Work out the finished part from the listing and answer in its coordinate system (mm). Face numbers are marked on the shaded views. Coordinates: 2 decimals unless noted, no trailing zeros. Write each loop counter-clockwise with the first axis right and the second up, starting at its lowest first coordinate (ties: lowest second). Pieces come first, ordered by that corner, then holes. Notation, with made-up numbers: (87, 79) - (94, 79) arc R15 ccw to (94, 96) - close; hole circle Ø3 at (59.5, 18.5). An arc over 180 degrees is marked (long way). Use one line per item in the form item = value. Start each with the question number.
Item 1: Consider probe 1 along X at (y, z) = (-6.5, -58.5); probe 2 along Z at (x, y) = (9, 2); probe 3 along Y at (x, z) = (-6.5, -59). Determine where each line is inside the solid, lowest interval first.
Item 2: A cutting plane is placed at B-B (z = 28.5). Write down the section's boundary in (x, y).
Item 3: A cutting plane is placed at A-A (x = 110.5). Write down the section's boundary in (y, z), then the cut area to 3 significant figures.
Item 4: Given pin 1 (1.6 mm diameter, centred on y = -7, z = -50.5, fed in from -X); pin 2 (1.6 mm diameter, centred on y = -7, z = -54, fed in from +X); pin 3 (5 mm diameter, centred on x = 30.5, y = 4, fed in from -Z), each flat-ended and moving along its own axis, determine where each tip first touches the part or whether it passes through.
Item 5: Determine the mould class of the marked faces 1 and 2 for opening direction X: released by +X, released by -X, zero draft, split by the parting line, or undercut.
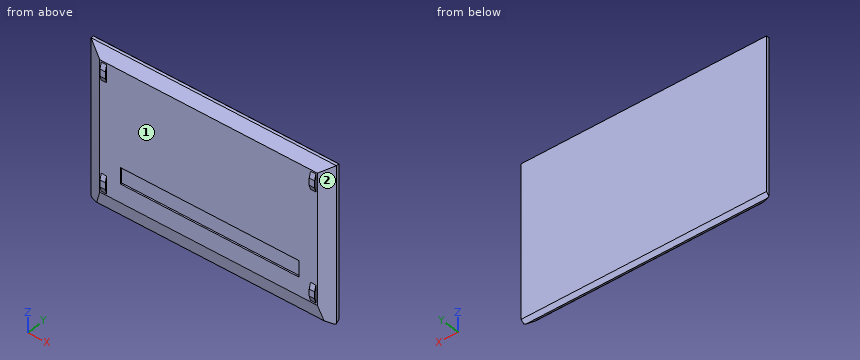
from build123d import *

# Parameters (mm, degrees)
BOSS_EXTRUDE2_DEPTH      = 160
CUT_EXTRUDE11_DEPTH      = 201.089979759
CUT_EXTRUDE11_DEPTH_BACK = 201.089979759
SKETCH12_W               = 233
SKETCH12_H               = 21
CUT_EXTRUDE12_DEPTH      = 2
SKETCH13_W               = 7
SKETCH13_H               = 23
BOSS_EXTRUDE3_DEPTH      = 2
CUT_EXTRUDE13_DEPTH      = 324.208910768
CUT_EXTRUDE13_DEPTH_BACK = 324.208910768


with BuildPart() as part:
    # Sketch8 → Boss-Extrude2 (new, symmetric)
    with BuildSketch(Plane(origin=(0, 0, 0), x_dir=(0, 0, -1), z_dir=(1, 0, 0))):
        Polygon((-88.104080333, -6), (62.895919667, -6), (80.895919667, -3.176729887), (80.976403784, -2.998472611), (82.781317846, 0.999074726), (78.781317846, 5.999074726), (-119.85604145, 6), (-120, 5.68), (-120, 1.998947428), (-106.104080333, -6), align=None)
    extrude(amount=BOSS_EXTRUDE2_DEPTH, both=True)

    # Sketch9 → Cut-Extrude11 (cut, two sides: drawn at the far end of the back side and taken through both)
    with BuildSketch(Plane.XY.offset(-CUT_EXTRUDE11_DEPTH_BACK)):
        Polygon((-160, -6), (-142, -6), (-160, 1.998947428), align=None)
        Polygon((160, -6), (142, -6), (160, 1.998947428), align=None)
    extrude(amount=CUT_EXTRUDE11_DEPTH + CUT_EXTRUDE11_DEPTH_BACK, mode=Mode.SUBTRACT)

    # Sketch12 → Cut-Extrude12 (cut)
    with BuildSketch(Plane.XZ.offset(6)):
        with Locations((1.5, -28.395919667)):
            Rectangle(SKETCH12_W, SKETCH12_H)
    extrude(amount=-CUT_EXTRUDE12_DEPTH, mode=Mode.SUBTRACT)

    # Sketch13 → Boss-Extrude3 (add)
    with BuildSketch(Plane.XZ.offset(6)):
        with Locations((-136.5, 92.604080333)):
            Rectangle(SKETCH13_W, SKETCH13_H)
        with Locations((-136.5, -49.395919667)):
            Rectangle(SKETCH13_W, SKETCH13_H)
        with Locations((136.5, -49.395919667)):
            Rectangle(SKETCH13_W, SKETCH13_H)
        with Locations((136.5, 92.604080333)):
            Rectangle(SKETCH13_W, SKETCH13_H)
    extrude(amount=BOSS_EXTRUDE3_DEPTH)

    # Sketch14 → Cut-Extrude13 (cut, two sides: drawn at the far end of the back side and taken through both)
    with BuildSketch(Plane.ZY.offset(140).offset(-CUT_EXTRUDE13_DEPTH_BACK)):
        Polygon((-60.895919667, -8), (-54.223413834, -8), (-60.895919667, -6), align=None)
        Polygon((104.104080333, -8), (96.367273939, -8), (104.104080333, -6), align=None)
        Polygon((81.104080333, -8), (81.104080333, -6), (87.367273939, -8), align=None)
        Polygon((-45.223413834, -8), (-37.895919667, -6), (-37.895919667, -8), align=None)
    extrude(amount=CUT_EXTRUDE13_DEPTH + CUT_EXTRUDE13_DEPTH_BACK, mode=Mode.SUBTRACT)


solid = part.part
Answer:
q1.probe_1 = -140 to -133, 133 to 140
q1.probe_2 = -81.98 to 120
q1.probe_3 = -6 to 6
q2.outline = (-160, 2) - (-142, -6) - (142, -6) - (160, 2) - (160, 6) - (-160, 6) - close
q3.outline = (-6, -62.9) - (-3.18, -80.9) - (1, -82.78) - (6, -78.78) - (6, 119.86) - (5.68, 120) - (2, 120) - (-6, 106.1) - (-6, -17.9) - (-4, -17.9) - (-4, -38.9) - (-6, -38.9) - close
q3.area = 2,290 mm²
q4.pin_1 = -140
q4.pin_2 = 140
q4.pin_3 = -82.38
q5.face_1 = undercut
q5.face_2 = released by +X
